The listing builds one solid part. Answer for the finished solid, in the listing's coordinates (mm). Round coordinates to 2 decimals unless told otherwise and drop trailing zeros. Write each loop counter-clockwise with the first axis right and the second up, starting at its lowest first coordinate (ties: lowest second). Pieces come first, ordered by that corner, then holes.
from build123d import *

# Parameters (mm, degrees)
F0_W     = 152.4
F0_H     = 152.4
F1_DEPTH = 12.7


with BuildPart() as f1:
    # F0 (on Top) → F1 (new body)
    with BuildSketch(Plane.XY):
        with Locations((76.2, 76.2)):
            Rectangle(F0_W, F0_H)
        Polygon((16.345332, 24.800697), (25.316621, 15.811483), (16.345332, 6.822268), (7.368064, 15.805512), (7.374039, 15.811483), (7.368064, 15.817454), align=None, mode=Mode.SUBTRACT)
        Polygon((16.345333, 52.520424), (25.316622, 43.53121), (16.345333, 34.541995), (7.368065, 43.525238), (7.374041, 43.53121), (7.368065, 43.537181), align=None, mode=Mode.SUBTRACT)
        Polygon((55.959203, 15.811483), (55.965178, 15.805512), (46.98791, 6.822268), (38.016621, 15.811483), (46.98791, 24.800697), (55.965178, 15.817454), align=None, mode=Mode.SUBTRACT)
        Polygon((77.642446, 24.800697), (86.613735, 15.811483), (77.642446, 6.822268), (68.665178, 15.805512), (68.671153, 15.811483), (68.665178, 15.817454), align=None, mode=Mode.SUBTRACT)
        Polygon((108.285023, 6.822268), (99.313735, 15.811483), (108.285023, 24.800697), (117.262291, 15.817454), (117.256316, 15.811483), (117.262291, 15.805512), align=None, mode=Mode.SUBTRACT)
        Polygon((145.104813, 15.793557), (145.110789, 15.787586), (136.133521, 6.804342), (127.162232, 15.793557), (136.133521, 24.782771), (145.110789, 15.799528), align=None, mode=Mode.SUBTRACT)
        Polygon((55.959204, 43.53121), (55.965179, 43.525238), (46.987911, 34.541995), (38.016622, 43.53121), (46.987911, 52.520424), (55.965179, 43.537181), align=None, mode=Mode.SUBTRACT)
        Polygon((77.642447, 52.520424), (86.613736, 43.53121), (77.642447, 34.541995), (68.665179, 43.525238), (68.671154, 43.53121), (68.665179, 43.537181), align=None, mode=Mode.SUBTRACT)
        Polygon((108.285025, 34.541995), (99.313736, 43.53121), (108.285025, 52.520424), (117.262293, 43.537181), (117.256317, 43.53121), (117.262293, 43.525238), align=None, mode=Mode.SUBTRACT)
        Polygon((145.104815, 43.513284), (145.11079, 43.507312), (136.133522, 34.524069), (127.162233, 43.513284), (136.133522, 52.502498), (145.11079, 43.519255), align=None, mode=Mode.SUBTRACT)
        Polygon((16.345333, 83.289459), (25.316622, 74.300244), (16.345333, 65.31103), (7.368065, 74.294273), (7.374041, 74.300244), (7.368065, 74.306215), align=None, mode=Mode.SUBTRACT)
        Polygon((16.345333, 114.266112), (25.316622, 105.276898), (16.345333, 96.287683), (7.368065, 105.270927), (7.374041, 105.276898), (7.368065, 105.282869), align=None, mode=Mode.SUBTRACT)
        Polygon((25.316622, 136.045932), (16.345333, 127.056718), (7.368065, 136.039961), (7.374041, 136.045932), (7.368065, 136.051904), (16.345333, 145.035147), align=None, mode=Mode.SUBTRACT)
        Polygon((38.016622, 74.300244), (46.987911, 83.289459), (55.965179, 74.306215), (55.959204, 74.300244), (55.965179, 74.294273), (46.987911, 65.31103), align=None, mode=Mode.SUBTRACT)
        Polygon((68.665179, 74.306215), (77.642447, 83.289459), (86.613736, 74.300244), (77.642447, 65.31103), (68.665179, 74.294273), (68.671154, 74.300244), align=None, mode=Mode.SUBTRACT)
        Polygon((46.987911, 96.287683), (38.016622, 105.276898), (46.987911, 114.266112), (55.965179, 105.282869), (55.959204, 105.276898), (55.965179, 105.270927), align=None, mode=Mode.SUBTRACT)
        Polygon((77.642447, 114.266112), (86.613736, 105.276898), (77.642447, 96.287683), (68.665179, 105.270927), (68.671154, 105.276898), (68.665179, 105.282869), align=None, mode=Mode.SUBTRACT)
        Polygon((108.285025, 65.31103), (99.313736, 74.300244), (108.285025, 83.289459), (117.262293, 74.306215), (117.256317, 74.300244), (117.262293, 74.294273), align=None, mode=Mode.SUBTRACT)
        Polygon((136.133522, 65.328956), (127.162233, 74.31817), (136.133522, 83.307385), (145.11079, 74.324141), (145.104815, 74.31817), (145.11079, 74.312199), align=None, mode=Mode.SUBTRACT)
        Polygon((108.285025, 114.266112), (117.262293, 105.282869), (117.256317, 105.276898), (117.262293, 105.270927), (108.285025, 96.287683), (99.313736, 105.276898), align=None, mode=Mode.SUBTRACT)
        Polygon((136.133522, 114.248186), (145.11079, 105.264943), (145.104815, 105.258972), (145.11079, 105.253001), (136.133522, 96.269757), (127.162233, 105.258972), align=None, mode=Mode.SUBTRACT)
        Polygon((46.987911, 127.056718), (38.016622, 136.045932), (46.987911, 145.035147), (55.965179, 136.051904), (55.959204, 136.045932), (55.965179, 136.039961), align=None, mode=Mode.SUBTRACT)
        Polygon((77.642447, 127.056718), (68.665179, 136.039961), (68.671154, 136.045932), (68.665179, 136.051904), (77.642447, 145.035147), (86.613736, 136.045932), align=None, mode=Mode.SUBTRACT)
        Polygon((108.285025, 127.056718), (99.313736, 136.045932), (108.285025, 145.035147), (117.262293, 136.051904), (117.256317, 136.045932), (117.262293, 136.039961), align=None, mode=Mode.SUBTRACT)
        Polygon((136.133522, 127.074644), (127.162233, 136.063858), (136.133522, 145.053073), (145.11079, 136.06983), (145.104815, 136.063858), (145.11079, 136.057887), align=None, mode=Mode.SUBTRACT)
    extrude(amount=F1_DEPTH)


solid = f1.part
1. Straight lines are drawn through the part: line 1 along X through (y, z) = (18.5, 8); line 2 along Y through (x, z) = (131, 6); line 3 along X through (y, z) = (77.5, 4.25). For each, find the intervals that lie inside material, in ascending order.
Geometry says:
line 1: x = 0 to 10.05, 22.63 to 40.7, 53.28 to 71.35, 83.93 to 102, 114.58 to 129.86, 142.41 to 152.4
line 2: y = 0 to 11.95, 19.64 to 39.67, 47.36 to 70.47, 78.16 to 101.41, 109.1 to 132.22, 139.91 to 152.4
line 3: x = 0 to 10.56, 22.12 to 41.21, 52.77 to 71.86, 83.42 to 102.51, 114.07 to 130.34, 141.94 to 152.4
2. Section A-A on x = 113.5 is taken. Determine the outline of the cut face in (y, z).
Geometry says:
outline: (0, 0) - (12.04, 0) - (12.04, 12.7) - (0, 12.7) - close; (19.58, 0) - (39.76, 0) - (39.76, 12.7) - (19.58, 12.7) - close; (47.3, 0) - (70.53, 0) - (70.53, 12.7) - (47.3, 12.7) - close; (78.07, 0) - (101.51, 0) - (101.51, 12.7) - (78.07, 12.7) - close; (109.05, 0) - (132.28, 0) - (132.28, 12.7) - (109.05, 12.7) - close; (139.82, 0) - (152.4, 0) - (152.4, 12.7) - (139.82, 12.7) - close
3. Section C-C on z = 3 is taken. Give the number of separate pieces and of enclosed holes in the cut face, plus the area to 3 significant figures.
Geometry says:
separate pieces: 1
enclosed holes: 25
area: 19,200 mm2
4. For a pull along X with two mould halves and no side action, classify faces 1 (the face through (103.862, 38.974, 6.261)), 2 (the face through (75, 94, 0)) as released by +X, released by -X, zero draft, split by the parting line, or undercut.
Geometry says:
face 1: undercut
face 2: zero draft
5. Section B-B on y = 50.5 is taken. Determine the outline of the cut face in (x, z).
Geometry says:
outline: (0, 0) - (14.33, 0) - (14.33, 12.7) - (0, 12.7) - close; (18.36, 0) - (44.97, 0) - (44.97, 12.7) - (18.36, 12.7) - close; (49.01, 0) - (75.62, 0) - (75.62, 12.7) - (49.01, 12.7) - close; (79.66, 0) - (106.27, 0) - (106.27, 12.7) - (79.66, 12.7) - close; (110.3, 0) - (134.14, 0) - (134.14, 12.7) - (110.3, 12.7) - close; (138.13, 0) - (152.4, 0) - (152.4, 12.7) - (138.13, 12.7) - close
